```python
from build123d import *

# Parameters (mm, degrees)
F0_R      = 35.9948936704
F1_DEPTH  = 25.4
F3_T      = -2.54
F5_DEPTH  = 25.401
F6_R      = 6.3781739211
F7_DEPTH  = 2.54
F9_DEPTH  = 114
F10_W     = 18.6832621694
F10_H     = 6.5605333075
F11_DEPTH = 114
F13_DEPTH = 114
F15_DEPTH = 114
F17_DEPTH = 25.401
F19_DEPTH = 35.9958936704
F20_R     = 3.0085790952
F21_DEPTH = 25.4
F22_R     = 2.5711256323
F23_DEPTH = 25.4


# Not quite as in the source:
# - an extrude ends at something that could not be found from the text; its depth is read off the source's solid


with BuildPart() as f1:
    # F0 (on Front) → F1 (new body)
    with BuildSketch(Plane.XZ):
        Circle(F0_R)
    extrude(amount=F1_DEPTH)

    # F3
    f3_openings = [f1.faces().sort_by_distance(p)[0] for p in [
        (0, -25.4, 0),
    ]]
    offset(amount=F3_T, openings=f3_openings)

    # F4 (on face) → F5 (cut, through all)
    with BuildSketch(Plane.XZ.offset(25.4)):
        Polygon((-13.4063111618, 12.1227279305), (-22.8192508221, 0), (-5.9900530614, 0), align=None)
    extrude(amount=-F5_DEPTH, mode=Mode.SUBTRACT)

    # F6 (on Front) → F7 (cut, through all)
    with BuildSketch(Plane.XZ):
        with Locations((11.409625411, 10.9817655757)):
            Circle(F6_R)
    extrude(amount=F7_DEPTH, mode=Mode.SUBTRACT)

    # F8 (on Front) → F9 (cut, through all)
    with BuildSketch(Plane.XZ):
        Polygon((7.8015748957, -15.0106055726), (4.1785330897, -8.0938870023), (-3.623041806, -7.7731739601), (-7.8015748957, -14.3691794883), (-4.1785330897, -21.2858980586), (3.623041806, -21.6066111008), align=None)
    extrude(amount=-F9_DEPTH, mode=Mode.SUBTRACT)

    # F10 (on Front) → F11 (cut, through all)
    with BuildSketch(Plane.XZ):
        with Locations((-9.3416310847, -10.1260426454)):
            Rectangle(F10_W, F10_H)
    extrude(amount=-F11_DEPTH, mode=Mode.SUBTRACT)

    # F12 (on Front) → F13 (cut, through all)
    with BuildSketch(Plane.XZ):
        Polygon((-16.4013374597, -20.2520862222), (12.4079678208, -20.2520862222), (14.9751342833, -13.9767900109), (-16.4013374597, -13.9767900109), align=None)
    extrude(amount=-F13_DEPTH, mode=Mode.SUBTRACT)

    # F14 (on Front) → F15 (cut, through all)
    with BuildSketch(Plane.XZ):
        Polygon((8.4161829098, -14.604808726), (4.1344067188, -7.3587224255), (-4.281776191, -7.4438062299), (-8.4161829098, -14.7749763349), (-4.1344067188, -22.0210626354), (4.281776191, -21.935978831), align=None)
    extrude(amount=-F15_DEPTH, mode=Mode.SUBTRACT)

    # F16 (on Front) → F17 (cut, through all)
    with BuildSketch(Plane.XZ):
        Polygon((5.7048136368, -15.7016435097), (5.7048136368, -9.1142921319), (0, -5.820616443), (-5.7048136368, -9.1142921319), (-5.7048136368, -15.7016435097), (0, -18.9953191986), align=None)
    extrude(amount=F17_DEPTH, mode=Mode.SUBTRACT)

    # F18 (on Top) → F19 (cut, through all)
    with BuildSketch(Plane.XY):
        Polygon((39.3632091582, -15.2603751048), (-36.7960445583, -15.5456149951), (-36.7960445583, -24.6733147651), (39.3632091582, -24.6733147651), align=None)
    extrude(amount=-F19_DEPTH, mode=Mode.SUBTRACT)

    # F20 (on Front) → F21 (join)
    with BuildSketch(Plane.XZ):
        with Locations((-36.7960445583, 0)):
            Circle(F20_R)
    extrude(amount=F21_DEPTH)

    # F22 (on Front) → F23 (join)
    with BuildSketch(Plane.XZ):
        with Locations((36.6534218192, 0)):
            Circle(F22_R)
    extrude(amount=F23_DEPTH)


solid = f1.part
```
Input: part model. Units: mm. Frame: model coordinates. A direction names the side the tool comes from. Coordinates: 2 decimals unless noted, no trailing zeros. Loops run counter-clockwise (first coordinate to the right, second up) from the corner with the lowest first, then second, coordinate; pieces in that order, holes last. Notation, with made-up numbers: M -29.75,-32.5 L 19.25,-32.5 A29 ccw 19.25,-0.5 Z; hole C 87.5,28.25 d2. An arc over 180 degrees is marked long. Answer in a Markdown table with one row per item.
1. Material intervals for line 1 (Z direction, x = 0, y = -4); line 2 (Y direction, x = -28, z = -14.5); line 3 (X direction, y = -7.5, z = 0), sorted ascending.
Response:
| item | result |
|---|---|
| line 1 | z = -35.99 to -33.45, 33.45 to 35.99 |
| line 2 | y = -2.54 to 0 |
| line 3 | x = -39.8 to -33.45, 33.45 to 39.22 |
2. Section B-B, the plane x = 25.5. Output: boundary loops of the cut face in (y, z), then the cut area to 3 significant figures.
Response:
| item | result |
|---|---|
| outline | M -25.4,-25.4 L -24.67,-25.4 L -24.67,-21.66 L -25.4,-21.66 Z; M -25.4,21.66 L -2.54,21.66 L -2.54,-21.66 L -15.31,-21.66 L -15.31,-25.4 L 0,-25.4 L 0,25.4 L -25.4,25.4 Z |
| area | 265 mm2 |
3. First-contact query: pin 1 (1 mm diameter, centred on y = -6.5, z = 26.5, fed in from +X); pin 2 (5 mm diameter, centred on x = 5, y = -20.5, fed in from -Z); pin 3 (6 mm diameter, centred on y = -18.5, z = 28.5, fed in from +X). Flat tips, straight axial feed; report the tip coordinate or a pass-through.
Response:
| item | result |
|---|---|
| pin 1 | stops at x = 24.89 |
| pin 2 | stops at z = 32.6 |
| pin 3 | stops at x = 25.4 |
4. Reachability of faces 1 (the flat face through (-18.047, -1.288, 6.146)), 2 (the flat face through (-1, 0, 1)), 3 (the cylindrical face through (-4.36, -11.27, 33.17)) from +Z, -Z, +X, -X, +Y, -Y: full face, straight path, thin tool, end or side. Return the list, or none.
Response:
| item | result |
|---|---|
| face 1 | +Y, -Y |
| face 2 | +Z, -Z, +X, -X, +Y |
| face 3 | -Y |
5. Section A-A, the plane z = -17. Output: boundary loops of the cut face in (x, y), then the cut area to 3 significant figures.
Response:
| item | result |
|---|---|
| outline | M -31.73,-25.4 L -28.81,-25.4 L -28.81,-24.67 L -31.73,-24.67 Z; M -31.73,-15.53 L -28.81,-15.52 L -28.81,-2.54 L -3.46,-2.54 L -3.46,0 L -31.73,0 Z; M 3.46,-2.54 L 28.81,-2.54 L 28.81,-15.3 L 31.73,-15.29 L 31.73,0 L 3.46,0 Z; M 28.81,-25.4 L 31.73,-25.4 L 31.73,-24.67 L 28.81,-24.67 Z |
| area | 223 mm2 |
6. Draft query along X for faces 4 (the flat face through (-33, -25.4, -8)), 5 (the flat face through (0, -2.54, 0)). Return one class per face: pulls with the +X half, pulls with the -X half, needs draft (parallel to the pull), parting line crosses it, or undercut.
Response:
| item | result |
|---|---|
| face 4 | needs draft |
| face 5 | undercut |
7. Section D-D, the plane z = 20. Output: boundary loops of the cut face in (x, y), then the cut area to 3 significant figures.
Response:
| item | result |
|---|---|
| outline | M -29.93,-25.4 L -26.82,-25.4 L -26.82,-2.54 L 26.82,-2.54 L 26.82,-25.4 L 29.93,-25.4 L 29.93,0 L -29.93,0 Z |
| area | 294 mm2 |
